from build123d import *

# Parameters (mm, degrees)
F1_DEPTH = 6.35
F0_R     = 17.314711
F2_DEPTH = 25.4
F3_DEPTH = 25.4


with BuildPart() as f1:
    # F0 (on Top) → F1 (new body)
    with BuildSketch(Plane.XY):
        with BuildLine():
            Line((-28.557787, 28.316794), (-28.557787, -5.904352))
            Line((-28.557787, -5.904352), (27.187924, -5.904352))
            ThreePointArc((27.187924, -5.904352), (23.335338, -0.750448), (20.958387, 5.229121))
            Line((20.958387, 5.229121), (-4.677194, 5.229121))
            Line((-4.677194, 5.229121), (-4.579983, 18.536286))
            Line((-4.579983, 18.536286), (21.340561, 18.536286))
            ThreePointArc((21.340561, 18.536286), (23.687391, 23.771415), (27.187924, 28.316794))
            Line((27.187924, 28.316794), (-28.557787, 28.316794))
        make_face()
    extrude(amount=F1_DEPTH)

    # F0 (on Top) → F2 (join)
    with BuildSketch(Plane.XY):
        with BuildLine():
            ThreePointArc((20.958387, 5.229121), (23.335338, -0.750448), (27.187924, -5.904352))
            ThreePointArc((27.187924, -5.904352), (53.942294, -11.471062), (69.191078, 11.206221))
            ThreePointArc((69.191078, 11.206221), (53.942294, 33.883504), (27.187924, 28.316794))
            ThreePointArc((27.187924, 28.316794), (23.687391, 23.771415), (21.340561, 18.536286))
            ThreePointArc((21.340561, 18.536286), (20.227784, 11.909174), (20.958387, 5.229121))
        make_face()
        with Locations((44.704385, 11.206221)):
            Circle(F0_R, mode=Mode.SUBTRACT)
    extrude(amount=F2_DEPTH)

    # F0 (on Top) → F3 (join)
    with BuildSketch(Plane.XY):
        with BuildLine():
            Line((-4.677194, 5.229121), (20.958387, 5.229121))
            ThreePointArc((20.958387, 5.229121), (20.227784, 11.909174), (21.340561, 18.536286))
            Line((21.340561, 18.536286), (-4.579983, 18.536286))
            Line((-4.579983, 18.536286), (-4.677194, 5.229121))
        make_face()
    extrude(amount=F3_DEPTH)


solid = f1.part
Read the model definition and answer for the solid it produces. Units are mm, in the model's axes. A direction names the side the tool comes from. Coordinates: 2 decimals unless noted, no trailing zeros. Write each loop counter-clockwise with the first axis right and the second up, starting at its lowest first coordinate (ties: lowest second). Pieces come first, ordered by that corner, then holes. Notation, with made-up numbers: (-10, -15) - (46, -15) arc R13 cw to (46, 1) - close; hole circle Ø9 at (-30, 51). An arc over 180 degrees is marked (long way). One line per question, with ' | ' between items.
Q1. Find section A-A, the plane x = 14. Write down the section's boundary in (y, z).
Result set:
outline: (-5.9, 0) - (28.32, 0) - (28.32, 6.35) - (18.54, 6.35) - (18.54, 25.4) - (5.23, 25.4) - (5.23, 6.35) - (-5.9, 6.35) - close
Q2. For faces 4 (the flat face through (-1, -5.904, 3)), 5 (the flat face through (0, 28.317, 3)), 6 (the flat face through (9, 18.536, 16)), determine the directions among +Z, -Z, +X, -X, +Y, -Y from which every point of the face is accessible in a straight line to the end or side of a thin tool.
Result set:
face 4: +Z, -Z, -X, -Y | face 5: +Z, -Z, -X, +Y | face 6: +Z, -X, +Y
Q3. Find section C-C, the plane y = 14. Write down the section's boundary in (x, z).
Result set:
outline: (-28.56, 0) - (27.62, 0) - (27.62, 25.4) - (-4.61, 25.4) - (-4.61, 6.35) - (-28.56, 6.35) - close; (61.79, 0) - (69.03, 0) - (69.03, 25.4) - (61.79, 25.4) - close
Q4. Each of these flat-tipped pins is pushed along its axis until it touches: P1, Ø7, axis at x = 0, z = 4, coming from the +Y side; P2, Ø3, axis at x = 11.5, z = 4.5, coming from the -Y side; P3, Ø21, axis at x = 44.7, y = 11.21, coming from the -Z side; P4, Ø8, axis at y = 17, z = 21.5, coming from the +X side. Where does it stop, or does it pass through?
Result set:
P1: y = 28.32 | P2: y = -5.9 | P3: through | P4: x = 69.13
Q5. Find section D-D, the plane x = 44.5. Write down the section's boundary in (y, z).
Result set:
outline: (-13.28, 0) - (-6.11, 0) - (-6.11, 25.4) - (-13.28, 25.4) - close; (28.52, 0) - (35.69, 0) - (35.69, 25.4) - (28.52, 25.4) - close
Q6. Determine the mould class of faces 1 (the flat face through (8, 5.229, 16)), 2 (the flat face through (9, 12, 0)), 3 (the cylindrical face through (61.22, 16.41, 12.52)) for opening direction Y: +Y half, -Y half, draft (parallel to the pull), parting line (faces both ways), or undercut.
Result set:
face 1: -Y half | face 2: draft | face 3: undercut
Q7. Find section B-B, the plane z = 23. Write down the section's boundary in (x, y), plus the area to 3 significant figures.
Result set:
outline: (-4.68, 5.23) - (20.96, 5.23) arc R24.49 ccw to (27.19, -5.9) arc R24.49 ccw (long way) to (27.19, 28.32) arc R24.49 ccw to (21.34, 18.54) - (-4.58, 18.54) - close; hole circle Ø34.63 at (44.7, 11.21) | area: 1,280 mm^2
Q8. Consider L1, parallel to Y at x = 44, z = 8; L2, parallel to X at y = 11, z = 4.5; L3, parallel to X at y = 4.5, z = 3. Determine where each line is inside the solid, lowest interval first. Write a range as [from, to].
Result set:
L1: [-13.27, -6.09], [28.51, 35.68] | L2: [-28.56, 27.39], [62.02, 69.19] | L3: [-28.56, 28.74], [60.67, 68.25]
